Drawing for the job (mm, zero at the part's lowest x, y, z). Coordinates: 2 decimals unless noted, no trailing zeros. Loops run counter-clockwise (first coordinate to the right, second up) from the corner with the lowest first, then second, coordinate; pieces in that order, holes last. Notation, with made-up numbers: (-22, -12) - (0, -12) arc R31 ccw to (0, 21) - close; hole circle Ø6 at (82, -35). An arc over 180 degrees is marked (long way). One line per item, written item: value.
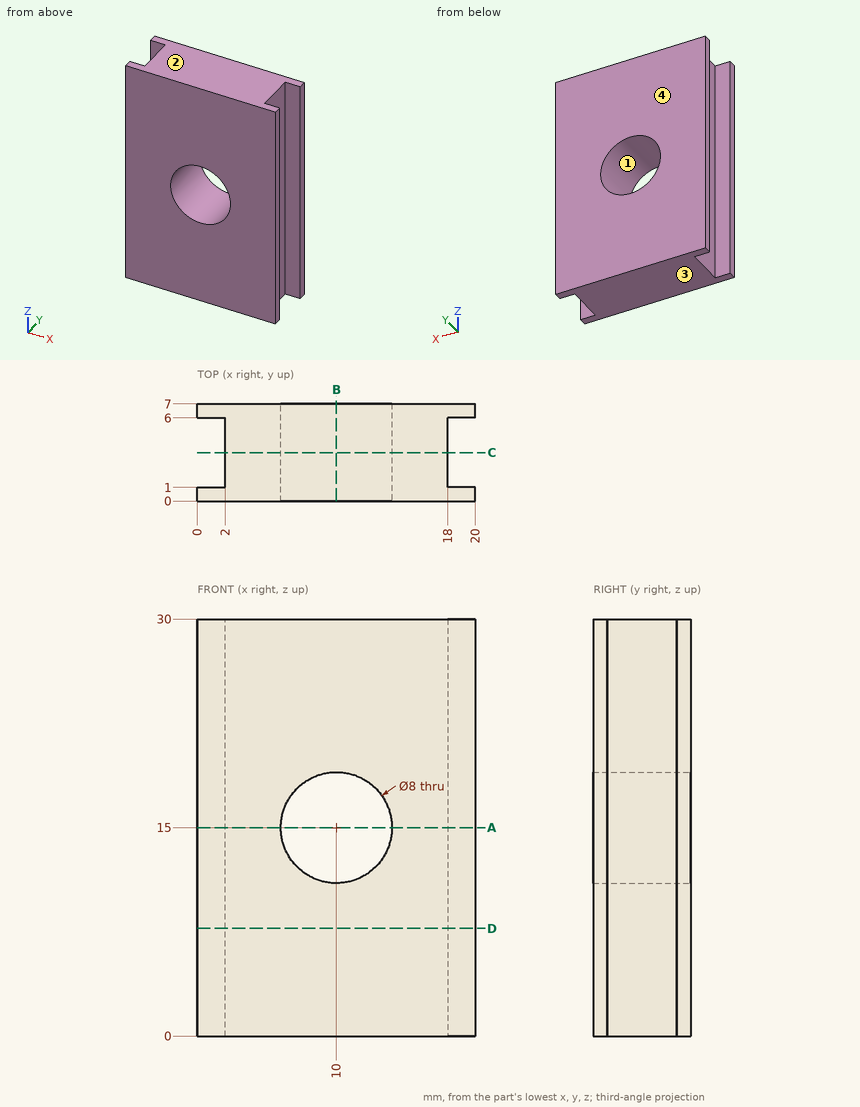
Item 1: Probe probe 1 along Y at (x, z) = (1.75, 25.75); probe 2 along Z at (x, y) = (10, 2); probe 3 along X at (y, z) = (5.25, 15). List the from-to ranges inside material, lowest first. Write a range as from..to.
Check result:
probe 1: y = 0..1, 6..7
probe 2: z = 0..11, 19..30
probe 3: x = 2..6, 14..18
Item 2: Cut at B-B, the plane x = 10. Write the cut outline in (y, z), then the cut area to 3 significant figures.
Check result:
outline: (0, 0) - (7, 0) - (7, 11) - (0, 11) - close; (0, 19) - (7, 19) - (7, 30) - (0, 30) - close
area: 154 mm^2
Item 3: Cut at A-A, the plane z = 15. Write the cut outline in (x, y), then the cut area to 3 significant figures.
Check result:
outline: (0, 0) - (6, 0) - (6, 7) - (0, 7) - (0, 6) - (2, 6) - (2, 1) - (0, 1) - close; (14, 0) - (20, 0) - (20, 1) - (18, 1) - (18, 6) - (20, 6) - (20, 7) - (14, 7) - close
area: 64.0 mm^2
Item 4: Cut at D-D, the plane z = 7.75. Write the cut outline in (x, y), then the cut area to 3 significant figures.
Check result:
outline: (0, 0) - (20, 0) - (20, 1) - (18, 1) - (18, 6) - (20, 6) - (20, 7) - (0, 7) - (0, 6) - (2, 6) - (2, 1) - (0, 1) - close
area: 120 mm^2
Item 5: Drop flat-ended pins along their axis: P1, Ø2.5, axis at y = 3.5, z = 12.5, coming from the +X side; P2, Ø2.5, axis at y = 3, z = 20.5, coming from the -X side. Give the stop position or say it passes through.
Check result:
P1: stops at x = 18
P2: stops at x = 2
Item 6: Cut at C-C, the plane y = 3.5. Write the cut outline in (x, z), then the cut area to 3 significant figures.
Check result:
outline: (2, 0) - (18, 0) - (18, 30) - (2, 30) - close; hole circle Ø8 at (10, 15)
area: 430 mm^2
Item 7: Pull direction Z, two halves, no side cores. Call the marked faces 1, 2, 3 and 4: released by +Z, released by -Z, zero draft, split by the parting line, or undercut.
Check result:
face 1: undercut
face 2: released by +Z
face 3: released by -Z
face 4: zero draft
